Could you check a few things on this model? Use its own coordinates, in mm. Coordinates: 2 decimals unless noted, no trailing zeros. Order: outer loops, then holes, each group sorted by start corner. A loop starts at its lowest first (then second) coordinate and runs counter-clockwise, first axis right, second up. Notation, with made-up numbers: (56.5, 33) - (62.5, 33) arc R18 ccw to (62.5, 49) - close; hole circle Ø9 at (6, 35.25). An arc over 180 degrees is marked (long way). One line per item, written item: value. Start each with the question number.
from build123d import *

# Parameters (mm, degrees)
EXTRUDE_1_DEPTH          = 4
PATTERN_CIRCULAR_1_COUNT = 20
CUT_EXTRUDE_1_DEPTH      = 19.538608362
CUT_EXTRUDE_1_DEPTH_BACK = 19.538608362
SKETCH_2_R               = 2.55


with BuildPart() as part:
    # 스케치1 → 보스-돌출1 (new body)
    with BuildSketch(Plane(origin=(0, 0, 0), x_dir=(0, 0, -1), z_dir=(1, 0, 0))):
        with BuildLine():
            ThreePointArc((0, 12.8), (1.158685544, 11.536663611), (1.578481404, 9.874633991))
            ThreePointArc((1.578481404, 9.874633991), (0, -10), (-1.578481404, 9.874633991))
            ThreePointArc((-1.578481404, 9.874633991), (-1.158685544, 11.536663611), (0, 12.8))
        make_face()
    extrude_1 = extrude(amount=EXTRUDE_1_DEPTH)

    # 원형 패턴1: 보스-돌출1 ×20 about axis
    pattern_circular_1_axis = Axis((0, 0, 0), (1, 0, 0))
    for i in range(1, PATTERN_CIRCULAR_1_COUNT):
        add(extrude_1.rotate(pattern_circular_1_axis, i * 360 / PATTERN_CIRCULAR_1_COUNT))

    # 스케치2 → 컷-돌출1 (cut, two sides: drawn at the far end of the back side and taken through both)
    with BuildSketch(Plane.ZY.offset(-CUT_EXTRUDE_1_DEPTH_BACK)):
        Circle(SKETCH_2_R)
    extrude(amount=CUT_EXTRUDE_1_DEPTH + CUT_EXTRUDE_1_DEPTH_BACK, mode=Mode.SUBTRACT)


solid = part.part
Q1. I want a section at B-B on y = -1.25. Please give me the cut outline in (x, z) (3 decimals).
Q2. I want a section at C-C on z = -0.5. Please give me the cut outline in (x, y), then the cut area to 3 significant figures.
Q3. If I drill on L1, parallel to Y at x = 1.5, z = 11; L2, parallel to Z at x = 2.7, y = 9.25; L3, parallel to Y at x = 3.85, z = 0.5, over which ranges is the centre line in solid material (lowest first)?
Q4. I want a section at D-D on y = -6. Please give me the cut outline in (x, z).
Q5. I'm going to push flat-ended pins straight in: pin 1 (1.5 mm diameter, centred on x = 3.5, y = 3, fed in from -Z); pin 2 (2 mm diameter, centred on x = 1.5, z = 10, fed in from +Y); pin 3 (1 mm diameter, centred on y = -4.5, z = 7.5, fed in from -X); pin 4 (4.5 mm diameter, centred on y = 0, z = 0, fed in from +X). Where does each tip first touch, or does it pass through?
Q6. I want a section at A-A on z = -9.5. Please give me the cut outline in (x, y), then the cut area to 3 significant figures.
Values follow:
1. outline: (0, -11.355) - (4, -11.355) - (4, -2.223) - (0, -2.223) - close; (0, 2.223) - (4, 2.223) - (4, 11.355) - (0, 11.355) - close
2. outline: (0, -12.4) - (4, -12.4) - (4, -2.5) - (0, -2.5) - close; (0, 2.5) - (4, 2.5) - (4, 12.4) - (0, 12.4) - close
2. area: 79.2 mm^2
3. L1: y = -4.57 to -2.16, -1.39 to 1.39, 2.16 to 4.57
3. L2: z = -7.75 to -4.8, -4.65 to 4.65, 4.8 to 7.75
3. L3: y = -12.4 to -2.5, 2.5 to 12.4
4. outline: (0, -10.08) - (4, -10.08) - (4, 10.08) - (0, 10.08) - close
5. pin 1: stops at z = -12.11
5. pin 2: stops at y = 7.75
5. pin 3: stops at x = 0
5. pin 4: passes through
6. outline: (0, -7.73) - (4, -7.73) - (4, -5.06) - (0, -5.06) - close; (0, -4.69) - (4, -4.69) - (4, 4.69) - (0, 4.69) - close; (0, 5.06) - (4, 5.06) - (4, 7.73) - (0, 7.73) - close
6. area: 58.9 mm^2
